Could you check a few things on this model? Use its own coordinates, in mm. A direction names the side the tool comes from. Give positions to 0.01 mm unless a question says otherwise; leave off trailing zeros. Order: outer loops, then holes, each group sorted by start corner. A loop starts at its lowest first (then second) coordinate and runs counter-clockwise, first axis right, second up. Notation, with made-up numbers: (-16, -16.5) - (4, -16.5) arc R21 cw to (4, -4.5) - close; hole circle Ø3 at (41, -23). An arc over 180 degrees is marked (long way). One line per question, with ' | ' between items. Start each with the question number.
1. Which directions (+Z, -Z, +X, -X, +Y, -Y) give clear straight access to the entire face, cutting with the end or side of a thin tool? Please do faces 4 (the cylindrical face through (-4.38, 38.67, -8.43)), 5 (the flat face through (0, 0, -7)), 6 (the flat face through (3.11, 1, -32)).
2. For P1, Ø12, axis at x = 14, z = -14, coming from the +Y side; P2, Ø3, axis at x = -6.5, y = 58.5, coming from the +Z side; P3, Ø6, axis at x = 3, z = -19, coming from the -Y side, each with a flat end and sliding along its axis, tell me the tip position at first contact or that it passes through.
3. Imagine slicing it at A-A (y = 38.5). Please give me the cut outline in (x, z), and give its area (3 significant figures).
4. I need wall thicknesses on probe 1 along Z at (x, y) = (0, 14.25); probe 2 along Y at (x, z) = (8, 11); probe 3 along Y at (x, z) = (-24.5, 24). Which ranges of each line are inside material? Lowest first, please. Write a range as from..to.
5. If we mould it in two halves opening along Z, with no side actions, what happens to faces 1 (the conical face through (-32.96, 7.204, 10.38)), 2 (the flat face through (0, 70.85, 0)), 3 (the cylindrical face through (2.58, 9.63, -0.81))? For each: released by +Z, released by -Z, zero draft, split by the parting line, or undercut.
```python
from build123d import *

# Parameters (mm, degrees)
CHAMFER1_SIZE               = 0.75
CHAMFER2_SIZE               = 3
CHAMFER2_SIZE2              = 5.196152423
F_1_4_28_TAPPED_HOLE2_D     = 5.4102
F_1_4_28_TAPPED_HOLE2_DEPTH = 19
F_1_4_28_TAPPED_HOLE2_TIP   = 1.625388061


with BuildPart() as part:
    # Sketch1 → Revolve1 (revolve)
    with BuildSketch(Plane.XY):
        Polygon((0, 0), (0, 70.85), (-9.5, 70.85), (-9.5, 7.35), (-39.5, 7.35), (-39.5, 1), (-32, 1), (-32, 0), align=None)
    revolve(axis=Axis((0, 0, 0), (0, 1, 0)))

    # Chamfer1
    chamfer1_edges = [part.edges().sort_by_distance(p)[0] for p in [
        (9.5, 7.35, 0),
        (9.5, 70.85, 0),
    ]]
    chamfer(chamfer1_edges, length=CHAMFER1_SIZE)

    # Chamfer2
    chamfer2_edges = [part.edges().sort_by_distance(p)[0] for p in [
        (39.5, 7.35, 0),
    ]]
    chamfer2_side = [part.faces().sort_by_distance(p)[0] for p in [
        (39.5, 4.175, 0),
    ]]
    chamfer(chamfer2_edges, length=CHAMFER2_SIZE, length2=CHAMFER2_SIZE2, reference=chamfer2_side[0])

    # 1/4-28 Tapped Hole2
    with Locations(Plane(origin=(0, 0, 0), x_dir=(-1, 0, 0), z_dir=(0, -1, 0))):
        with Locations((86.483740344, -12.823451155), (0, 0)):
            Hole(F_1_4_28_TAPPED_HOLE2_D / 2, depth=F_1_4_28_TAPPED_HOLE2_DEPTH)
            with Locations((0, 0, -(F_1_4_28_TAPPED_HOLE2_DEPTH + F_1_4_28_TAPPED_HOLE2_TIP / 2))):  # 118° drill point
                Cone(0, F_1_4_28_TAPPED_HOLE2_D / 2, F_1_4_28_TAPPED_HOLE2_TIP, mode=Mode.SUBTRACT)


solid = part.part
```
Results found:
1) face 4: +Y | face 5: +Z, -Z, +X, -X, -Y | face 6: -Y
2) P1: stops at y = 7.35 | P2: stops at z = 8.08 | P3: stops at y = 0
3) outline: circle Ø19 at (0, 0) | area: 284 mm2
4) probe 1: z = -9.5..-2.71, 2.71..9.5 | probe 2: y = 0..7.35 | probe 3: y = 1..7.35
5) face 1: split by the parting line | face 2: zero draft | face 3: undercut
